Part model, mm, in its own coordinate system. A direction names the side the tool comes from. Give positions to 0.01 mm unless a question says otherwise; leave off trailing zeros. Write each loop counter-clockwise with the first axis right and the second up, starting at its lowest first coordinate (ties: lowest second). Pieces come first, ordered by that corner, then holes. Notation, with made-up numbers: (-22, 16.5) - (10, 16.5) arc R15 ccw to (10, 45.5) - close; hole circle Ø9 at (73.5, 29). An arc over 180 degrees is marked (long way). Answer in a Markdown table with one row per item. Add a question column.
1. Band-saw the part on C-C on x = -6.25. Write the cut outline in (y, z), plus the area to 3 significant figures.
2. Pull direction Z, two halves, no side cores. Call faces 3 (the flat face through (2, -5, 124.1)), 4 (the flat face through (0, 0, 128)), 5 (the flat face through (0, 0, 0)): released by +Z, released by -Z, zero draft, split by the parting line, or undercut.
3. Drop flat-ended pins along their axis: pin 1 Ø8 at (x, y) = (-1, -1.5) entering from -Z; pin 2 Ø4 at (y, z) = (2.5, 103.5) entering from +X; pin 3 Ø4 at (x, z) = (-2.5, 19) entering from +Y; pin 4 Ø3 at (y, z) = (4, 98) entering from +X. Give the stop position or say it passes through.
4. Which spindle directions (+Z, -Z, +X, -X, +Y, -Y) get a long thin tool onto all of the face, cutting with end or side? Do faces 1 (the cylindrical face through (-7.493, 0.33, 126.023)), 2 (the cylindrical face through (-1.08, -4.88, 63.16)). Say none if no direction does.
5. Probe line 1 along Z through (x, y) = (5.25, 4.75); line 2 along Y through (x, z) = (-0.5, 119.5). List the from-to ranges inside material, lowest first.
6. Band-saw the part on A-A on y = 0. Write the cut outline in (x, z).
7. Band-saw the part on D-D on z = 40.5. Write the cut outline in (x, y).
```python
from build123d import *

# Parameters (mm, degrees)
SKETCH1_R           = 7.5
SKETCH1_R_2         = 5
BOSS_EXTRUDE1_DEPTH = 128
CUT_EXTRUDE1_START  = 3.9
SKETCH1_6_R         = 7.5
SKETCH1_6_R_2       = 5
CUT_EXTRUDE1_DEPTH  = 120.2


with BuildPart() as part:
    # Sketch1 → Boss-Extrude1 (new body)
    with BuildSketch(Plane.XY):
        Circle(SKETCH1_R)
        Circle(SKETCH1_R_2, mode=Mode.SUBTRACT)
        Circle(SKETCH1_R_2)
    extrude(amount=BOSS_EXTRUDE1_DEPTH)

    # Sketch1<6> → Cut-Extrude1 (cut)
    with BuildSketch(Plane.XY.offset(CUT_EXTRUDE1_START)):
        Circle(SKETCH1_6_R)
        Circle(SKETCH1_6_R_2, mode=Mode.SUBTRACT)
    extrude(amount=CUT_EXTRUDE1_DEPTH, mode=Mode.SUBTRACT)


solid = part.part
```
Values:
| question | item | result |
|---|---|---|
| 1 | outline | (-4.15, 0) - (4.15, 0) - (4.15, 3.9) - (-4.15, 3.9) - close; (-4.15, 124.1) - (4.15, 124.1) - (4.15, 128) - (-4.15, 128) - close |
| 1 | area | 64.7 mm² |
| 2 | face 3 | undercut |
| 2 | face 4 | released by +Z |
| 2 | face 5 | released by -Z |
| 3 | pin 1 | stops at z = 0 |
| 3 | pin 2 | stops at x = 4.97 |
| 3 | pin 3 | stops at y = 4.97 |
| 3 | pin 4 | stops at x = 4.33 |
| 4 | face 1 | +Z, -Z |
| 4 | face 2 | none |
| 5 | line 1 | z = 0 to 3.9, 124.1 to 128 |
| 5 | line 2 | y = -4.97 to 4.97 |
| 6 | outline | (-7.5, 0) - (7.5, 0) - (7.5, 3.9) - (5, 3.9) - (5, 124.1) - (7.5, 124.1) - (7.5, 128) - (-7.5, 128) - (-7.5, 124.1) - (-5, 124.1) - (-5, 3.9) - (-7.5, 3.9) - close |
| 7 | outline | circle Ø10 at (0, 0) |
